Autodesk Inventor part; units mm, degrees
ref_plane "YZ Plane" through (0, 0, 0) normal (1, 0, 0) x (0, 1, 0)
ref_plane "XZ Plane" through (0, 0, 0) normal (0, 1, 0) x (-1, 0, 0)
ref_plane "XY Plane" through (0, 0, 0) normal (0, 0, 1) x (1, 0, 0)
sketch "Sketch1" plane through (0, 0, 0) normal (0, 0, 1) x (1, 0, 0)
  circle A0 centre (0, 0) radius 4.85
  dimension "d0" = 9.7
extrude "Extrusion1" add sketch "Sketch1" against normal blind 7.84
sketch "Sketch2" plane through (0, 0, -7.84) normal (0, 0, -1) x (-1, 0, 0)
  circle A0 centre (0, 0) radius 4.85
  circle A1 centre (0, 0) radius 3.65
  circle A2 centre (0, 0) radius 4.85
  dimension "d3" = 7.3
extrude "Extrusion2" cut sketch "Sketch2" against normal blind 2.6
sketch "Sketch5" plane through (0, 0, -7.84) normal (0, 0, -1) x (-1, 0, 0)
  circle A0 centre (0, 0) radius 2.7
  dimension "d21" = 5.4
extrude "Extrusion4" cut sketch "Sketch5" against normal blind 6
sketch "Sketch6" plane through (0, 0, -1.84) normal (0, 0, -1) x (-1, 0, 0)
  circle A0 centre (0, 0) radius 2.25
  dimension "d24" = 4.5
extrude "Extrusion5" cut sketch "Sketch6" against normal through all
sketch "Sketch7" plane through (0, 0, 0) normal (1, 0, 0) x (0, 1, 0)
  line L0 (4.85, 1) -> (4.85, -1.3)
  arc A0 (4.85, -1.3) -> (2.25, -1.3) centre (3.55, -1.3) ccw
  line L1 (2.25, -1.3) -> (2.25, 1)
  line L2 (2.25, 1) -> (4.85, 1)
  line L3 (0, 6.9365) -> (0, -11.7629) construction
  point P0 (0, 0)
  point P1 (4.85, -0.15)
  dimension "d27" = 4.85
  dimension "d28" = 2.25
  dimension "d29" = 1.3
  dimension "d30" = 1
revolve "Revolution2" cut sketch "Sketch7" angle 360 about axis through (0, 0, 6.9365) along (0, 0, -1)
chamfer "Chamfer2" distance 0.2 angle 45 1 edges at (-4.85, 0, -5.24)
properties part number "cap_top"
The listing builds one solid part. Answer for the finished solid, in the listing's coordinates (mm). A direction names the side the tool comes from. Give positions to 0.01 mm unless a question says otherwise; leave off trailing zeros. Write each loop counter-clockwise with the first axis right and the second up, starting at its lowest first coordinate (ties: lowest second). Pieces come first, ordered by that corner, then holes.
1) Section A-A (y = 0) is taken. Write down the section's boundary in (x, z).
2) Section C-C (z = -3) is taken. Write down the section's boundary in (x, y).
3) Find the intervals of material crossed by L1, parallel to Y at x = 0, z = -3.45; L2, parallel to X at y = 0, z = -1.55; L3, parallel to Y at x = 0, z = -6, in increasing order.
4) Section D-D (z = -6) is taken. Write down the section's boundary in (x, y), and give its area (3 significant figures).
5) Given P1, Ø2, axis at y = -2.5, z = -5.5, coming from the +X side; P2, Ø1.5, axis at y = -2, z = -4, coming from the +X side; P3, Ø1.5, axis at x = -2, y = -3.5, coming from the -Z side; P4, Ø2.5, axis at x = -1, y = 1, coming from the -Z side, each flat-ended and moving along its own axis, determine where each tip first touches the part or whether it passes through.
6) For a pull along X with two mould halves and no side action, classify faces 1 (the face through (0.585, -2.636, -4.882)), 2 (the face through (-3, 0, -7.84)), 3 (the face through (-3.48, 1.1, -6.56)), 4 (the face through (0.29, 2.23, -1.57)) as pulls with the +X half, pulls with the -X half, needs draft (parallel to the pull), parting line crosses it, or undercut.
7) A tool of negligible diameter and unlimited length cuts with its end or side. For faces 5 (the face through (4.626, 1.457, -3.144)), 6 (the face through (0, -4, -5.24)), from which of +Z, -Z, +X, -X, +Y, -Y can it reach the whole face along a straight path? Write none if from no direction.
Response:
1. outline: (-4.85, -5.04) - (-4.65, -5.24) - (-3.65, -5.24) - (-3.65, -7.84) - (-2.7, -7.84) - (-2.7, -1.84) - (-2.25, -1.84) - (-2.25, -1.3) arc R1.3 ccw to (-4.85, -1.3) - close; (2.25, -1.84) - (2.7, -1.84) - (2.7, -7.84) - (3.65, -7.84) - (3.65, -5.24) - (4.65, -5.24) - (4.85, -5.04) - (4.85, -1.3) arc R1.3 ccw to (2.25, -1.3) - close
2. outline: circle Ø9.7 at (0, 0); hole circle Ø5.4 at (0, 0)
3. L1: y = -4.85 to -2.7, 2.7 to 4.85
3. L2: x = -4.85 to -2.25, 2.25 to 4.85
3. L3: y = -3.65 to -2.7, 2.7 to 3.65
4. outline: circle Ø7.3 at (0, 0); hole circle Ø5.4 at (0, 0)
4. area: 19.0 mm2
5. P1: stops at x = 4.57
5. P2: stops at x = 4.69
5. P3: stops at z = -7.84
5. P4: stops at z = -1.84
6. face 1: undercut
6. face 2: needs draft
6. face 3: parting line crosses it
6. face 4: undercut
7. face 5: +Z, -Z
7. face 6: -Z
